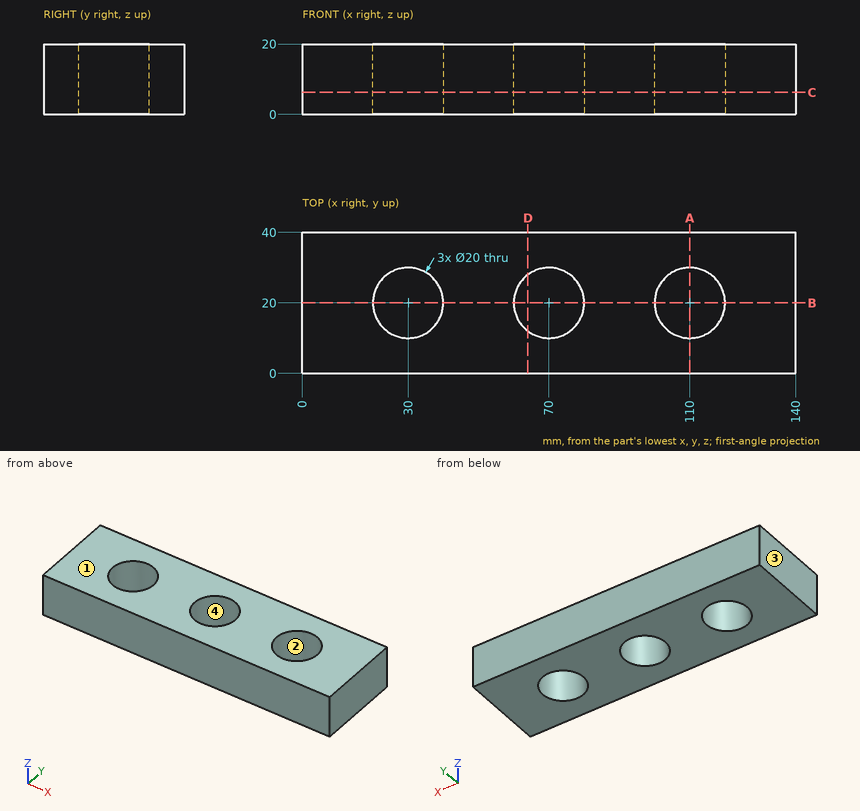
Input: dimensioned drawing with shaded views. Units: mm. Origin: part minimum x, y, z. Coordinates: 2 decimals unless noted, no trailing zeros. Loops run counter-clockwise (first coordinate to the right, second up) from the corner with the lowest first, then second, coordinate; pieces in that order, holes last. Notation, with made-up numbers: (70, 26.5) - (117, 26.5) arc R27 cw to (117, 54.5) - close; hole circle Ø2 at (-39, 64). An arc over 180 degrees is marked (long way). One line per question, with ' | ' between items. Start each with the question number.
(1) Cut plane B-B on y = 20. Output: boundary loops of the cut face in (x, z), and give its area (3 significant figures).
(2) Draft query along X for the marked faces 1, 2, 3 and 4. Return one class per face: +X half, -X half, draft (parallel to the pull), parting line (faces both ways), or undercut.
(3) First-contact query: pin 1 (1.5 mm diameter, centred on x = 24, z = 6, fed in from -Y); pin 2 (12 mm diameter, centred on x = 70, y = 20, fed in from -Z). Flat tips, straight axial feed; report the tip coordinate or a pass-through.
(4) Cut plane D-D on x = 64. Output: boundary loops of the cut face in (y, z).
(5) Ray query, L1, parallel to Y at x = 110, z = 10.75; L2, parallel to X at y = 12, z = 1.5; L3, parallel to X at y = 13.5, z = 5.75. Return the intervals inside material, ascending. Write a range as from..to.
(6) Cut plane C-C on z = 6.25. Output: boundary loops of the cut face in (x, y).
(7) Cut plane A-A on x = 110. Output: boundary loops of the cut face in (y, z).
Here are the results:
1) outline: (0, 0) - (20, 0) - (20, 20) - (0, 20) - close; (40, 0) - (60, 0) - (60, 20) - (40, 20) - close; (80, 0) - (100, 0) - (100, 20) - (80, 20) - close; (120, 0) - (140, 0) - (140, 20) - (120, 20) - close | area: 1,600 mm²
2) face 1: draft | face 2: undercut | face 3: -X half | face 4: undercut
3) pin 1: y = 0 | pin 2: through
4) outline: (0, 0) - (12, 0) - (12, 20) - (0, 20) - close; (28, 0) - (40, 0) - (40, 20) - (28, 20) - close
5) L1: 0..10, 30..40 | L2: 0..24, 36..64, 76..104, 116..140 | L3: 0..22.4, 37.6..62.4, 77.6..102.4, 117.6..140
6) outline: (0, 0) - (140, 0) - (140, 40) - (0, 40) - close; hole circle Ø20 at (30, 20); hole circle Ø20 at (70, 20); hole circle Ø20 at (110, 20)
7) outline: (0, 0) - (10, 0) - (10, 20) - (0, 20) - close; (30, 0) - (40, 0) - (40, 20) - (30, 20) - close
